Geometry: final body of the model. Coordinates: model frame, mm. Face numbers are marked on the shaded views. A direction names the side the tool comes from. Coordinates: 2 decimals unless noted, no trailing zeros. One line per item, written item: value. Start each with the question number.
Item 1: Mould query, pull axis X, two halves, no side actions, for the marked faces 1, 2 and 3. Classes: +X half, -X half, draft (parallel to the pull), parting line (faces both ways), or undercut.
Item 2: Set-up query: the marked faces 4 and 5. Return all of +Z, -Z, +X, -X, +Y, -Y with unobstructed straight access to the full face (end or side cutting, diameter ignored); none if empty.
Item 3: Ray query, probe 1 along Z at (x, y) = (-7, -8.25); probe 2 along X at (y, z) = (-6.8, 4.5); probe 3 along Z at (x, y) = (-7, -9.55). Return the intervals inside material, ascending. Write a range as from..to.
Item 4: Contact query for flat-ended pins moving along their axis: pin 1 Ø1.7 at (x, z) = (5, 1.5) entering from -Y; pin 2 Ø3.5 at (x, y) = (3.5, 3.5) entering from +Z; pin 3 Ø1 at (x, z) = (-15.5, 91.5) entering from +Y. Output: stop coordinate, or through.
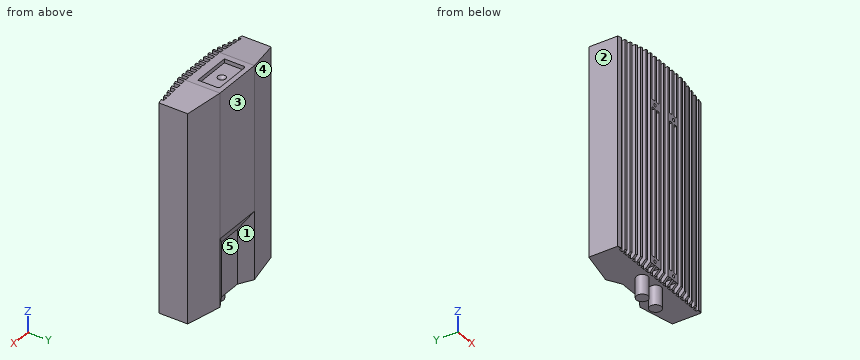
from build123d import *

# Parameters (mm, degrees)
EXTRUDE_1_DEPTH        = 109.5
SKETCH_2_W             = 26
SKETCH_2_H             = 50
CUT_EXTRUDE_1_DEPTH    = 4
CUT_EXTRUDE_1_DRAFT    = -60
CUT_EXTRUDE_2_DEPTH    = 127.786483901
CUT_EXTRUDE_3_DEPTH    = 116.951498481
CUT_EXTRUDE_4_DEPTH    = 2
SKETCH_7_W             = 6.8
SKETCH_7_H             = 4
EXTRUDE_2_DEPTH        = 3.5
HOLE_WIZARD_M2_1_D     = 1.6
HOLE_WIZARD_M2_1_DEPTH = 5.2
HOLE_WIZARD_M2_1_TIP   = 0.480688495
SKETCH_11_R            = 3
EXTRUDE_3_DEPTH        = 10


with BuildPart() as part:
    # 草图1 → 凸台-拉伸1 (new body)
    with BuildSketch(Plane.XY):
        Polygon((31.5, 6.75), (31.5, -8.25), (29.05, -8.581081081), (29.05, -7.25), (26.95, -7.25), (26.95, -8.864864865), (25.75, -9.027027027), (25.75, -7.25), (23.65, -7.25), (23.65, -9.310810811), (22.45, -9.472972973), (22.45, -7.25), (20.35, -7.25), (20.35, -9.756756757), (19.15, -9.918918919), (19.15, -7.25), (17.05, -7.25), (17.05, -10.202702703), (15.85, -10.364864865), (15.85, -7.25), (13.75, -7.25), (13.75, -10.648648649), (13, -10.75), (12.55, -10.75), (12.55, -7.25), (10.45, -7.25), (10.45, -10.75), (9.25, -10.75), (9.25, -7.25), (7.15, -7.25), (7.15, -10.75), (5.95, -10.75), (5.95, -7.25), (3.85, -7.25), (3.85, -10.75), (2.65, -10.75), (2.65, -7.25), (0.55, -7.25), (0.55, -10.75), (-0.55, -10.75), (-0.55, -7.25), (-2.65, -7.25), (-2.65, -10.75), (-3.85, -10.75), (-3.85, -7.25), (-5.95, -7.25), (-5.95, -10.75), (-7.15, -10.75), (-7.15, -7.25), (-9.25, -7.25), (-9.25, -10.75), (-10.45, -10.75), (-10.45, -7.25), (-12.55, -7.25), (-12.55, -10.75), (-13, -10.75), (-13.75, -10.648648649), (-13.75, -7.25), (-15.85, -7.25), (-15.85, -10.364864865), (-17.05, -10.202702703), (-17.05, -7.25), (-19.15, -7.25), (-19.15, -9.918918919), (-20.35, -9.756756757), (-20.35, -7.25), (-22.45, -7.25), (-22.45, -9.472972973), (-23.65, -9.310810811), (-23.65, -7.25), (-25.75, -7.25), (-25.75, -9.027027027), (-26.95, -8.864864865), (-26.95, -7.25), (-29.05, -7.25), (-29.05, -8.581081081), (-31.5, -8.25), (-31.5, 6.75), (-13, 10.75), (13, 10.75), align=None)
    extrude(amount=EXTRUDE_1_DEPTH)


with BuildPart() as cut_extrude_1_tool:
    # 草图2 → 切除-拉伸1 (with draft: the straight prism first)
    with BuildSketch(Plane(origin=(0, 10.75, 0), x_dir=(1, 0, 0), z_dir=(0, 1, 0))):
        with Locations((0, -10)):
            Rectangle(SKETCH_2_W, SKETCH_2_H)
    extrude(amount=-CUT_EXTRUDE_1_DEPTH)
    # 切除-拉伸1: the draft: its side faces are tilted about the plane it starts from
    cut_extrude_1_sides = [cut_extrude_1_tool.faces().sort_by_distance(p)[0] for p in [
        (-13, 8.75, 10),
        (0, 8.75, 35),
        (13, 8.75, 10),
        (0, 8.75, -15),
    ]]
    draft(cut_extrude_1_sides, Plane(origin=(0, 10.75, 0), x_dir=(1, 0, 0), z_dir=(0, 1, 0)), CUT_EXTRUDE_1_DRAFT)


with BuildPart() as part_1:
    add(part.part)

    # 切除-拉伸1: cut by cut_extrude_1_tool
    add(cut_extrude_1_tool.part, mode=Mode.SUBTRACT)

    # 草图3 → 切除-拉伸2 (cut, through all)
    with BuildSketch(Plane(origin=(31.5, 0, 0), x_dir=(0, 0, -1), z_dir=(1, 0, 0))):
        Polygon((0, -8.25), (-2.5, -10.75), (0, -10.75), align=None)
    extrude(amount=-CUT_EXTRUDE_2_DEPTH, mode=Mode.SUBTRACT)

    # 草图4 → 切除-拉伸3 (cut, through all)
    with BuildSketch(Plane(origin=(0, 10.75, 0), x_dir=(1, 0, 0), z_dir=(0, 1, 0))):
        Polygon((13, -109.5), (31.5, -107.5), (31.5, -109.5), align=None)
        Polygon((-31.5, -107.5), (-31.5, -109.5), (-13, -109.5), align=None)
    extrude(amount=-CUT_EXTRUDE_3_DEPTH, mode=Mode.SUBTRACT)

    # 草图5 → 切除-拉伸4 (cut)
    with BuildSketch(Plane.XY.offset(109.5)):
        with BuildLine():
            Line((-9, 8.25), (9, 8.25))
            ThreePointArc((9, 8.25), (9.707106781, 7.957106781), (10, 7.25))
            Line((10, 7.25), (10, -2.75))
            Line((10, -2.75), (-10, -2.75))
            Line((-10, -2.75), (-10, 7.25))
            ThreePointArc((-10, 7.25), (-9.707106781, 7.957106781), (-9, 8.25))
        make_face()
    extrude(amount=-CUT_EXTRUDE_4_DEPTH, mode=Mode.SUBTRACT)

    # 切除-拉伸5 cone 1 section (through the dimple's axis) → 切除-拉伸5 (revolve, cut)
    with BuildSketch(Plane(origin=(0, 2.75, 107.5), x_dir=(0, -1, 0), z_dir=(1, 0, 0))):
        Polygon((0, 0), (2, 0), (0, 1.154700538), align=None)
    revolve(axis=Axis((0, 2.75, 107.5), (0, 0, -1)), mode=Mode.SUBTRACT)

    # 草图7 → 凸台-拉伸2 (add)
    with BuildSketch(Plane.XZ.offset(10.75)):
        with Locations((-7, 84.5)):
            Rectangle(SKETCH_7_W, SKETCH_7_H)
        with Locations((7, 84.5)):
            Rectangle(SKETCH_7_W, SKETCH_7_H)
        with Locations((7, 4.5)):
            Rectangle(SKETCH_7_W, SKETCH_7_H)
        with Locations((-7, 4.5)):
            Rectangle(SKETCH_7_W, SKETCH_7_H)
    extrude(amount=-EXTRUDE_2_DEPTH)

    # M2 螺纹孔1
    with Locations(Plane(origin=(0, -10.75, 0), x_dir=(-1, 0, 0), z_dir=(0, -1, 0))):
        with Locations((7, -4.5), (-7, -4.5), (7, -84.5), (-7, -84.5)):
            Hole(HOLE_WIZARD_M2_1_D / 2, depth=HOLE_WIZARD_M2_1_DEPTH)
            with Locations((0, 0, -(HOLE_WIZARD_M2_1_DEPTH + HOLE_WIZARD_M2_1_TIP / 2))):  # 118° drill point
                Cone(0, HOLE_WIZARD_M2_1_D / 2, HOLE_WIZARD_M2_1_TIP, mode=Mode.SUBTRACT)

    # 草图11 → 凸台-拉伸3 (add)
    with BuildSketch(Plane(origin=(0, 0, 0), x_dir=(-1, 0, 0), z_dir=(0, 0, -1))):
        with Locations((5, -2.75)):
            Circle(SKETCH_11_R)
        with Locations((-5, -2.75)):
            Circle(SKETCH_11_R)
    extrude(amount=EXTRUDE_3_DEPTH)


solid = part_1.part
Reply:
1. face 1: undercut
1. face 2: -X half
1. face 3: draft
2. face 4: +Z, -Z, -X, +Y
2. face 5: -Z, +Y
3. probe 1: z = 0..3.7, 5.3..83.7, 85.3..109.5
3. probe 2: x = -31.5..-7.8, -6.2..6.2, 7.8..31.5
3. probe 3: z = 1.3..3.7, 5.3..83.7, 85.3..109.5
4. pin 1: stops at y = -7.25
4. pin 2: stops at z = 107.5
4. pin 3: stops at y = 10.32
